The figure shows three views and two pictorial views of one solid part (mm, origin at its lowest corner). Answer the questions. Give positions to 0.01 mm unless a question says otherwise; leave off trailing zeros. Write each loop counter-clockwise with the first axis right and the second up, starting at its lowest first coordinate (ties: lowest second). Pieces come first, ordered by that corner, then holes. Notation, with made-up numbers: (-4.75, -2) - (2.25, -2) arc R20 ccw to (2.25, 13) - close; hole circle Ø7 at (-4, -9). An arc over 180 degrees is marked (long way). Use CSV: the item, a comma, the result in double quotes. Start each with the question number.
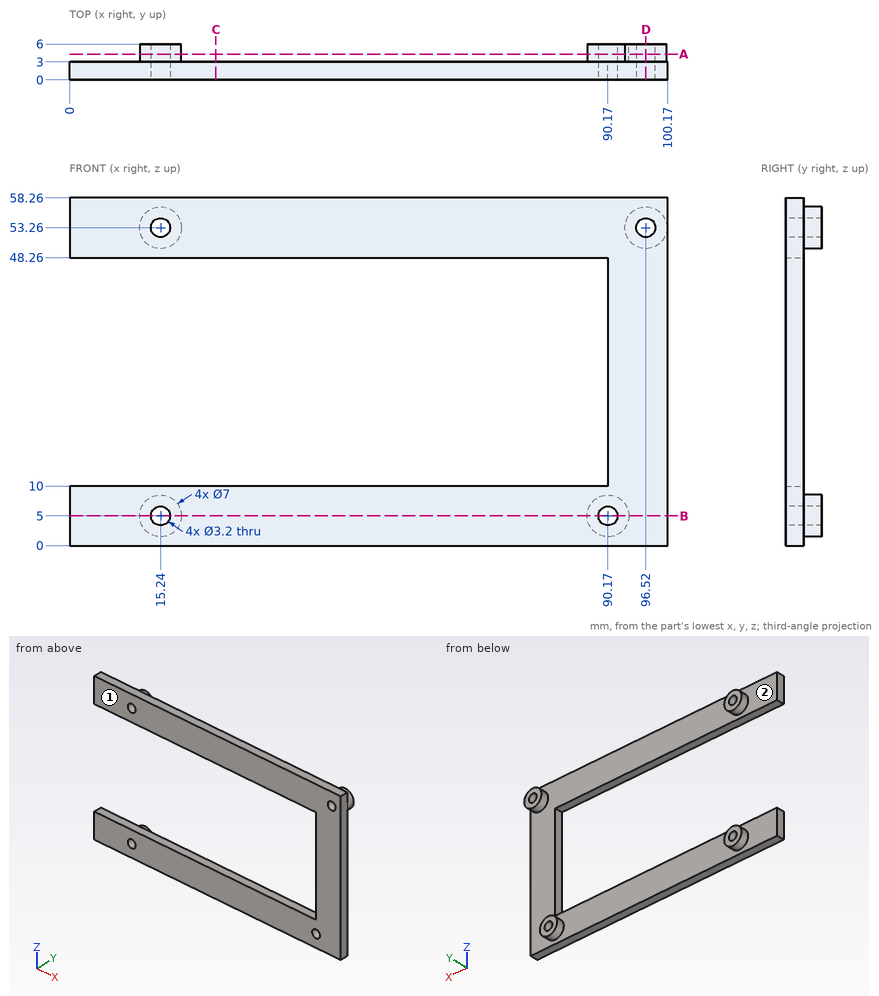
(1) Consider probe 1 along X at (y, z) = (4, 53.26); probe 2 along X at (y, z) = (2.9, 5); probe 3 along X at (y, z) = (3.95, 53). Determine where each line is inside the solid, lowest interval first.
(2) The part is cut by section C-C on x = 24.5. Write down the section's boundary in (y, z).
(3) The part is cut by section D-D on x = 96.52. Write down the section's boundary in (y, z).
(4) Given P1, Ø3.5, axis at x = 55, y = 2, coming from the -Z side; P2, Ø3.5, axis at y = 1, z = 25, coming from the -X side; P3, Ø8, axis at x = 65.5, z = 10, coming from the +Y side, each flat-ended and moving along its own axis, determine where each tip first touches the part or whether it passes through.
(5) For a pull along X with two mould halves and no side action, classify the marked faces 1 and 2 as pulls with the +X half, pulls with the -X half, needs draft (parallel to the pull), parting line crosses it, or undercut.
(6) The part is cut by section A-A on y = 4.3. Write down the section's boundary in (x, z).
(7) The part is cut by section B-B on z = 5. Write down the section's boundary in (x, y).
Reported:
1,probe 1,"11.74 to 13.64, 16.84 to 18.74, 93.02 to 94.92, 98.12 to 100.02"
1,probe 2,"0 to 13.64, 16.84 to 88.57, 91.77 to 100.17"
1,probe 3,"11.75 to 13.66, 16.82 to 18.73, 93.03 to 94.94, 98.1 to 100.01"
2,outline,"(0, 0) - (3, 0) - (3, 10) - (0, 10) - close; (0, 48.26) - (3, 48.26) - (3, 58.26) - (0, 58.26) - close"
3,outline,"(0, 0) - (3, 0) - (3, 49.76) - (6, 49.76) - (6, 51.66) - (0, 51.66) - close; (0, 54.86) - (6, 54.86) - (6, 56.76) - (3, 56.76) - (3, 58.26) - (0, 58.26) - close"
4,P1,"z = 0"
4,P2,"x = 90.17"
4,P3,"y = 3"
5,face 1,"needs draft"
5,face 2,"undercut"
6,outline,"circle Ø7 at (15.24, 5); circle Ø7 at (15.24, 53.26); circle Ø7 at (90.17, 5); circle Ø7 at (96.52, 53.26); hole circle Ø3.2 at (15.24, 5); hole circle Ø3.2 at (15.24, 53.26); hole circle Ø3.2 at (90.17, 5); hole circle Ø3.2 at (96.52, 53.26)"
7,outline,"(0, 0) - (13.64, 0) - (13.64, 6) - (11.74, 6) - (11.74, 3) - (0, 3) - close; (16.84, 0) - (88.57, 0) - (88.57, 6) - (86.67, 6) - (86.67, 3) - (18.74, 3) - (18.74, 6) - (16.84, 6) - close; (91.77, 0) - (100.17, 0) - (100.17, 3) - (93.67, 3) - (93.67, 6) - (91.77, 6) - close"
